```python
from build123d import *

# Parameters (mm, degrees)
SKETCH_1_W               = 30
SKETCH_1_H               = 28
EXTRUDE_1_DEPTH          = 6
SKETCH_2_R               = 1.75
CUT_EXTRUDE_1_DEPTH      = 7
SKETCH_4_R               = 2.75
CUT_EXTRUDE_4_DEPTH      = 3.5
CUT_EXTRUDE_4_DEPTH_BACK = 7
EXTRUDE_2_DEPTH          = 6
SKETCH_6_R               = 5
CUT_EXTRUDE_5_DEPTH      = 3.5
CHAMFER_1_SIZE           = 2
CUT_EXTRUDE_6_REACH      = 12
SKETCH_8_R               = 1.25


with BuildPart() as part:
    # 草图1 → 凸台-拉伸1 (new body)
    with BuildSketch(Plane(origin=(0, 0, 0), x_dir=(1, 0, 0), z_dir=(0, 1, 0))):
        Rectangle(SKETCH_1_W, SKETCH_1_H)
    extrude(amount=EXTRUDE_1_DEPTH)

    # 草图2 → 切除-拉伸1 (cut, through all)
    with BuildSketch(Plane(origin=(0, 6, 0), x_dir=(1, 0, 0), z_dir=(0, 1, 0))):
        with Locations((-5, 9.5)):
            Circle(SKETCH_2_R)
        with Locations((5, 9.5)):
            Circle(SKETCH_2_R)
        with Locations((-5, -9.5)):
            Circle(SKETCH_2_R)
        with Locations((5, -9.5)):
            Circle(SKETCH_2_R)
    extrude(amount=-CUT_EXTRUDE_1_DEPTH, mode=Mode.SUBTRACT)

    # 草图4 → 切除-拉伸4 (cut, two sides)
    with BuildSketch(Plane.XZ) as cut_extrude_4_sk:
        with Locations((-9, 0)):
            Circle(SKETCH_4_R)
        with Locations((9, 0)):
            Circle(SKETCH_4_R)
    extrude(amount=CUT_EXTRUDE_4_DEPTH, mode=Mode.SUBTRACT)
    extrude(cut_extrude_4_sk.sketch, amount=-CUT_EXTRUDE_4_DEPTH_BACK, mode=Mode.SUBTRACT)

    # 草图7 → 凸台-拉伸2 (add)
    with BuildSketch(Plane(origin=(0, 6, 0), x_dir=(1, 0, 0), z_dir=(0, 1, 0))):
        Polygon((15, 74), (15, 14), (5, 14), (5, 64), (5, 94), (15, 94), align=None)
    extrude(amount=-EXTRUDE_2_DEPTH)

    # 草图6 → 切除-拉伸5 (cut)
    with BuildSketch(Plane.XZ):
        with Locations((-9, 0)):
            Circle(SKETCH_6_R)
        with Locations((9, 0)):
            Circle(SKETCH_6_R)
    extrude(amount=-CUT_EXTRUDE_5_DEPTH, mode=Mode.SUBTRACT)

    # 倒角1
    chamfer_1_edges = [part.edges().sort_by_distance(p)[0] for p in [
        (5, 3, -94),
        (15, 3, -94),
        (15, 3, 14),
        (-15, 3, 14),
        (-15, 3, -14),
    ]]
    chamfer(chamfer_1_edges, length=CHAMFER_1_SIZE)

    # 草图8 → 切除-拉伸6 (cut, up to next)
    with BuildSketch(Plane.ZY.offset(-5), mode=Mode.PRIVATE) as cut_extrude_6_sk1:
        with Locations((-86, 3)):
            Circle(SKETCH_8_R)
    cut_extrude_6_tool1 = extrude(cut_extrude_6_sk1.sketch, amount=-CUT_EXTRUDE_6_REACH, mode=Mode.PRIVATE) & part.part
    add(cut_extrude_6_tool1.solids().sort_by_distance((5, 3, -86))[0], mode=Mode.SUBTRACT)


solid = part.part
```
Verification items for the finished model (mm, model axes). A direction names the side the tool comes from. Coordinates: 2 decimals unless noted, no trailing zeros. Order: outer loops, then holes, each group sorted by start corner. A loop starts at its lowest first (then second) coordinate and runs counter-clockwise, first axis right, second up. Notation, with made-up numbers: (30, -27) -> (71, -27) arc R27 ccw to (71, -4) -> close; hole circle Ø4 at (-20.5, 74). An arc over 180 degrees is marked (long way). Put each result on its own line as item: value. Start each with the question number.
1) Cross-section at D-D (z = -86). Enter the section's corners in (x, y), plus the area to 3 significant figures.
2) Cross-section at A-A (x = 9). Enter the section's corners in (y, z).
3) Go/stop test with flat-tipped pins: pin 1 (9 mm diameter, centred on x = 9, z = 0, fed in from -Y); pin 2 (1.5 mm diameter, centred on y = 3, z = -16.5, fed in from -X); pin 3 (1.8 mm diameter, centred on x = -1, y = 4.5, fed in from -Z). Record where each tip stops, or that it passes through.
4) Cross-section at C-C (z = -9.5). Enter the section's corners in (x, y).
5) Release check for a two-part mould opening along X. For faces 4 (the flat face through (15, 3, -39)), 5 (the flat face through (-6.8, 3.5, -2.2)), 6 (the flat face through (7, 0, -29)), 7 (the cylindrical face through (-5.228, 3.042, 7.765)) record: pulls with the +X half, pulls with the -X half, needs draft (parallel to the pull), parting line crosses it, or undercut.
6) Material ranges on L1, parallel to Z at x = 10, y = 2.65; L2, parallel to Z at x = 9, y = 1; L3, parallel to Z at x = 4, y = 5.75, recorded low to high.
7) Tool access check on faces 1 (the flat face through (5, 3, -54)), 2 (the flat face through (11.2, 3.5, -2.2)), 3 (the flat face through (14, 3, -93)). Record the directions out of +Z, -Z, +X, -X, +Y, -Y that give a thin tool (end or side, any length) a straight path to the whole face; none if there is none.
8) Cross-section at B-B (x = -5). Enter the section's corners in (y, z).
Geometry check:
1. outline: (5, 0) -> (15, 0) -> (15, 1.75) -> (5, 1.75) -> close; (5, 4.25) -> (15, 4.25) -> (15, 6) -> (5, 6) -> close
1. area: 35.0 mm^2
2. outline: (0, -94) -> (6, -94) -> (6, -2.75) -> (3.5, -2.75) -> (3.5, -5) -> (0, -5) -> close; (0, 5) -> (3.5, 5) -> (3.5, 2.75) -> (6, 2.75) -> (6, 14) -> (0, 14) -> close; hole circle Ø2.5 at (3, -86)
3. pin 1: stops at y = 3.5
3. pin 2: stops at x = 5
3. pin 3: stops at z = -14
4. outline: (-15, 0) -> (-6.75, 0) -> (-6.75, 6) -> (-15, 6) -> close; (-3.25, 0) -> (3.25, 0) -> (3.25, 6) -> (-3.25, 6) -> close; (6.75, 0) -> (15, 0) -> (15, 6) -> (6.75, 6) -> close
5. face 4: pulls with the +X half
5. face 5: undercut
5. face 6: needs draft
5. face 7: undercut
6. L1: z = -94 to -87.2, -84.8 to -4.9, 4.9 to 14
6. L2: z = -94 to -5, 5 to 14
6. L3: z = -14 to -10.94, -8.06 to 8.06, 10.94 to 14
7. face 1: -Z, -X, +Y, -Y
7. face 2: -Y
7. face 3: -Z, +X, +Y, -Y
8. outline: (0, -14) -> (6, -14) -> (6, -11.25) -> (0, -11.25) -> close; (0, -7.75) -> (6, -7.75) -> (6, 7.75) -> (0, 7.75) -> (0, 3) -> (3.5, 3) -> (3.5, -3) -> (0, -3) -> close; (0, 11.25) -> (6, 11.25) -> (6, 14) -> (0, 14) -> close
